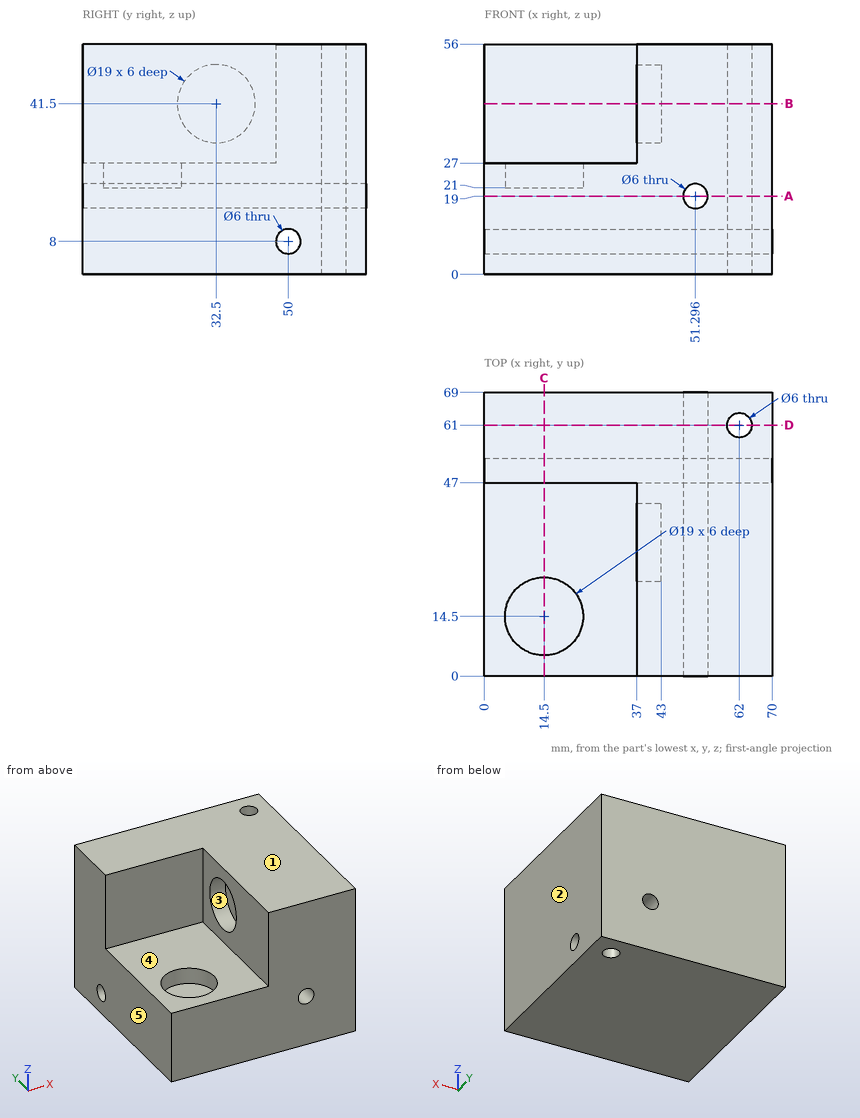
Design review of the part shown in the three views and the two pictorial views. Dimensions are in mm from the part's minimum x, y and z. A direction names the side the tool comes from. Give positions to 0.01 mm unless a question says otherwise; leave off trailing zeros. Write each loop counter-clockwise with the first axis right and the second up, starting at its lowest first coordinate (ties: lowest second). Pieces come first, ordered by that corner, then holes.
(1) Wall thickness on line 1 along Z through (x, y) = (58, 50); line 2 along Y through (x, z) = (38.5, 8); line 3 along Y through (x, z) = (14.5, 23.95): over which ranges is each line inside the solid? List them lowest first.
Checked values:
line 1: z = 0 to 5, 11 to 56
line 2: y = 0 to 47, 53 to 69
line 3: y = 0 to 5, 24 to 69
(2) Add section D-D (y = 61). Give the boundary of the cut face in (x, z).
Checked values:
outline: (0, 0) - (59, 0) - (59, 56) - (0, 56) - close; (65, 0) - (70, 0) - (70, 56) - (65, 56) - close; hole circle Ø6 at (51.3, 19)
(3) Add section C-C (x = 14.5). Give the boundary of the cut face in (y, z), and give its area (3 significant figures).
Checked values:
outline: (0, 0) - (69, 0) - (69, 56) - (47, 56) - (47, 27) - (24, 27) - (24, 21) - (5, 21) - (5, 27) - (0, 27) - close; hole circle Ø6 at (50, 8)
area: 2,360 mm2
(4) Clearance check with flat-ended pins moving along their axes: pin 1 Ø1.5 at (x, y) = (10.5, 9.5) entering from +Z; pin 2 Ø15 at (y, z) = (31.5, 38) entering from -X; pin 3 Ø23 at (y, z) = (33, 38) entering from -X; pin 4 Ø21 at (x, y) = (14.5, 11) entering from +Z. State where each tip first meets the part, or that it passes through.
Checked values:
pin 1: stops at z = 21
pin 2: stops at x = 37
pin 3: stops at x = 0
pin 4: stops at z = 27
(5) Tool access review of the marked faces 4 and 5: name each direction out of +Z, -Z, +X, -X, +Y, -Y from which nothing blocks a thin tool from reaching the whole face with its end or side.
Checked values:
face 4: +Z, -X, -Y
face 5: +Z, -Z, -X, +Y, -Y
(6) Mouldability with a two-part tool opening along Z and no side actions: class the marked faces 1, 2 and 3 as +Z half, -Z half, draft (parallel to the pull), parting line (faces both ways), or undercut.
Checked values:
face 1: +Z half
face 2: draft
face 3: undercut
(7) Add section A-A (z = 19). Give the boundary of the cut face in (x, y).
Checked values:
outline: (0, 0) - (48.3, 0) - (48.3, 69) - (0, 69) - close; (54.3, 0) - (70, 0) - (70, 69) - (54.3, 69) - close; hole circle Ø6 at (62, 61)
(8) Add section B-B (z = 41.5). Give the boundary of the cut face in (x, y).
Checked values:
outline: (0, 47) - (37, 47) - (37, 42) - (43, 42) - (43, 23) - (37, 23) - (37, 0) - (70, 0) - (70, 69) - (0, 69) - close; hole circle Ø6 at (62, 61)
